from build123d import *

# Parameters (mm, degrees)
F0_W      = 49.733065
F0_H      = 45.29678
F1_DEPTH  = 25.4
F1_FACE_W = 49.733066
F1_FACE_H = 45.29678
F2_DEPTH  = 12
F5_DEPTH  = 49.734065
F7_DEPTH  = 45.297781


with BuildPart() as f1:
    # F0 (on Top) → F1 (new body)
    with BuildSketch(Plane.XY):
        with Locations((2.985905, 5.489435)):
            Rectangle(F0_W, F0_H)
    extrude(amount=F1_DEPTH)

    # F1_face (on face) → F2 (join)
    with BuildSketch(Plane(origin=(2.985906, 5.489435, 25.4), x_dir=(1, 0, 0), z_dir=(0, 0, 1))):
        Rectangle(F1_FACE_W, F1_FACE_H)
    extrude(amount=F2_DEPTH)

    # F4 (on face) → F5 (cut, through all)
    with BuildSketch(Plane.YZ.offset(27.852438)):
        Polygon((10.376193, 15.41099), (10.376193, 8.385699), (19.320368, 0), (20.085741, 0), (19.943943, 2.660368), align=None)
    extrude(amount=-F5_DEPTH, mode=Mode.SUBTRACT)

    # F6 (on face) → F7 (cut, through all)
    with BuildSketch(Plane.XZ.offset(17.158955)):
        Polygon((6.854975, 6.713986), (4.791144, 2.940124), (8.41759, 0.257144), align=None)
    extrude(amount=-F7_DEPTH, mode=Mode.SUBTRACT)


solid = f1.part
For this review, take the finished solid that the model builds, in its own axes (mm). A direction names the side the tool comes from. Round coordinates to 2 decimals unless told otherwise and drop trailing zeros. Order: outer loops, then holes, each group sorted by start corner. A loop starts at its lowest first (then second) coordinate and runs counter-clockwise, first axis right, second up. Notation, with made-up numbers: M -34.75,42 L -20.75,42 A19 ccw -20.75,79 Z; hole C 52.25,-2.75 d6. An arc over 180 degrees is marked long. Use a Markdown table: item, result. Add a question column.
Item 1: Add section C-C, the plane z = 14. Give the boundary of the cut face in (x, y).
Item 2: Mouldability with a two-part tool opening along X and no side actions: class faces 1 (the flat face through (-21.881, 5, 31)), 2 (the flat face through (27.852, 5, 31)), 3 (the flat face through (5.838, 23.69, 4.853)), 4 (the flat face through (3.33, 14.79, 4.25)) as released by +X, released by -X, zero draft, split by the parting line, or undercut.
Item 3: To check wall thickness, follow line 1 along Y through (x, z) = (1, 2.5); line 2 along Z through (x, y) = (-14, 18.5); line 3 along X through (y, z) = (20.5, 2). State the ranges of each line that lie inside material, in increasing order.
Item 4: Insertion check: pin 1 (4 mm diameter, centred on x = 8.5, y = -7, fed in from -Z). The pin has a flat end and moves straight along its axis. Give the tip position at first contact, or say it passes through.
Item 5: Add section D-D, the plane z = 5. Give the boundary of the cut face in (x, y), then the cut area to 3 significant figures.
Item 6: Tool access review of faces 5 (the flat face through (3, 6, 37.4)), 6 (the flat face through (3.334, 20.016, 1.312)), 7 (the flat face through (3, 1, 0)), 8 (the flat face through (3.334, 15.227, 8.946)), 9 (the flat face through (7.647, 0.69, 3.44)): name each direction out of +Z, -Z, +X, -X, +Y, -Y from which nothing blocks a thin tool from reaching the whole face with its end or side.
Item 7: Add section A-A, the plane x = 9.5. Give the boundary of the cut face in (y, z).
Item 8: Add section B-B, the plane y = 11. State how many separate pieces and enclosed holes the cut face has, then the cut area to 3 significant figures.
Geometry results:
| question | item | result |
|---|---|---|
| 1 | outline | M -21.88,-17.16 L 27.85,-17.16 L 27.85,10.38 L -21.88,10.38 Z; M -21.88,11.43 L 27.85,11.43 L 27.85,28.14 L -21.88,28.14 Z |
| 2 | face 1 | released by -X |
| 2 | face 2 | released by +X |
| 2 | face 3 | undercut |
| 2 | face 4 | zero draft |
| 3 | line 1 | y = -17.16 to 16.65, 19.95 to 28.14 |
| 3 | line 2 | z = 0 to 0.77, 4.58 to 37.4 |
| 3 | line 3 | x = -21.88 to 6.06, 8 to 27.85 |
| 4 | pin 1 | stops at z = 0 |
| 5 | outline | M -21.88,-17.16 L 5.92,-17.16 L 5.92,13.99 L -21.88,13.99 Z; M -21.88,18.19 L 5.92,18.19 L 5.92,28.14 L -21.88,28.14 Z; M 7.27,-17.16 L 27.85,-17.16 L 27.85,13.99 L 7.27,13.99 Z; M 7.27,18.19 L 27.85,18.19 L 27.85,28.14 L 7.27,28.14 Z |
| 5 | area | 1,990 mm² |
| 6 | face 5 | +Z, +X, -X, +Y, -Y |
| 6 | face 6 | -Z, +X, -X |
| 6 | face 7 | -Z, +X, -X, +Y, -Y |
| 6 | face 8 | +X, -X |
| 6 | face 9 | +Y, -Y |
| 7 | outline | M -17.16,0 L 19.32,0 L 10.38,8.39 L 10.38,15.41 L 19.94,2.66 L 20.09,0 L 28.14,0 L 28.14,37.4 L -17.16,37.4 Z |
| 8 | separate pieces | 2 |
| 8 | enclosed holes | 1 |
| 8 | area | 1,510 mm² |
